Read the model definition and answer for the solid it produces. Units are mm, in the model's axes. A direction names the side the tool comes from. Coordinates: 2 decimals unless noted, no trailing zeros. Write each loop counter-clockwise with the first axis right and the second up, starting at its lowest first coordinate (ties: lowest second). Pieces come first, ordered by that corner, then holes.
(1) Which of the six approach directions +Z, -Z, +X, -X, +Y, -Y give full straight-line access (tool end or side, diameter ignored) to faces 4 (the flat face through (66.302, -3.639, 4.93)), 5 (the flat face through (-66.751, -3.898, 4.93)), 6 (the flat face through (-67.34, -39.36, 4.93))?
(2) Find the intervals of material crossed by probe 1 along Z at (x, y) = (59, 0); probe 2 along Y at (x, z) = (0, 7); probe 3 along Z at (x, y) = (-50, -10), in increasing order.
(3) Given pin 1 (12 mm diameter, centred on x = 25, z = 853.5, fed in from +Y); pin 2 (10 mm diameter, centred on y = 42.5, z = 256, fed in from -X); pin 3 (2 mm diameter, centred on x = 16, y = 53.5, fed in from +Z); pin 4 (1 mm diameter, centred on x = -12, y = 14, fed in from -Z), each flat-ended and moving along its own axis, determine where each tip first touches the part or whether it passes through.
(4) Section A-A on y = 25 is taken. Write down the section's boundary in (x, z), then the cut area to 3 significant figures.
(5) The mould has two halves that part along Z. Classify faces 1 (the flat face through (67.76, -38.64, 4.93)), 2 (the flat face through (-7, 5, 0)), 3 (the cylindrical face through (-57.887, -37.099, 1129.553)): +Z half, -Z half, draft (parallel to the pull), parting line (faces both ways), or undercut.
(6) Section B-B on z = 1074 is taken. Write down the section's boundary in (x, y).
Autodesk Inventor part; units mm, degrees
ref_plane "YZ Plane" through (0, 0, 0) normal (1, 0, 0) x (0, 1, 0)
ref_plane "XZ Plane" through (0, 0, 0) normal (0, 1, 0) x (-1, 0, 0)
ref_plane "XY Plane" through (0, 0, 0) normal (0, 0, 1) x (1, 0, 0)
sketch "Sketch1" plane through (0, 0, 0) normal (0, 0, 1) x (1, 0, 0)
  line L0 (-30, 78) -> (30, 78)
  line L1 (30, 78) -> (30, 8)
  line L2 (30, 8) -> (-30, 8)
  line L3 (-30, 8) -> (-30, 78)
  line L4 (119.0409, 377.068) -> (884.0572, 377.068) construction
  line L5 (884.0572, 377.068) -> (884.0572, -61.283) construction
  line L6 (884.0572, -61.283) -> (119.0409, -61.283) construction
  line L7 (119.0409, -61.283) -> (119.0409, 377.068) construction
  line L8 (528.2997, 310.003) -> (528.2997, 129.9198)
  line L9 (528.2997, 219.9614) -> (642.893, 286.807)
  circle A0 centre (0, 65) radius 6.5
  point P0 (0, 0)
  point P1 (0, 8)
  point P2 (0, 78)
  dimension "d9" = 60
  dimension "d10" = 70
  dimension "d13" = 78
  dimension "d14" = 13
  dimension "d15" = 13
extrude "Extrusion1" add sketch "Sketch1" along normal blind 10
pattern_circular "Circular Pattern1" count 3 over 360 about axis through (0, 0, -10) along (0, 0, 1) of "Extrusion1"
sketch "Sketch2" plane through (0, 0, 0) normal (0, 0, 1) x (1, 0, 0)
  circle A0 centre (0, 0) radius 50.8
  dimension "d21" = 101.6
extrude "Extrusion2" add sketch "Sketch2" along normal blind 1211
sketch "Sketch3" plane through (0, 0, 0) normal (1, 0, 0) x (0, 1, 0)
  circle A0 centre (0, 83) radius 48.75
  circle A1 centre (0, 83) radius 46.75
  point P0 (0, 0)
  dimension "d24" = 97.5
  dimension "d25" = 83
  dimension "d112" = 2
extrude "Extrusion3" add sketch "Sketch3" along normal blind 82.8
sketch "Sketch4" plane through (0, 0, 0) normal (1, 0, 0) x (0, 1, 0)
  circle A0 centre (0, 1158) radius 48.75
  line L0 (508.6061, 725.4056) -> (1697.4131, 725.4056) construction
  line L1 (1697.4131, 725.4056) -> (1697.4131, 178.9914) construction
  line L2 (1697.4131, 178.9914) -> (508.6061, 178.9914) construction
  line L3 (508.6061, 178.9914) -> (508.6061, 725.4056) construction
  line L4 (1437.8763, 515.5441) -> (1697.4131, 515.5441)
  line L5 (1697.4131, 515.5441) -> (1697.4131, 335.5441)
  line L6 (1697.4131, 335.5441) -> (1437.8763, 335.5441)
  line L7 (1437.8763, 335.5441) -> (1437.8763, 515.5441)
  line L8 (1526.1756, 486.7469) -> (1616.156, 486.7469)
  line L9 (40.9956, 0) -> (40.9956, 10)
  line L10 (40.9956, 0) -> (5.483, 0)
  line L11 (5.483, 10) -> (5.483, 0)
  line L12 (-46.4786, 10) -> (5.483, 10)
  line L13 (-46.4786, 0) -> (-46.4786, 10)
  line L14 (-46.4786, 0) -> (-46.4786, 0)
  line L15 (-46.4786, 10) -> (-46.4786, 0)
  line L16 (5.483, 10) -> (-46.4786, 10)
  line L17 (5.483, 0) -> (5.483, 10)
  line L18 (5.483, 0) -> (40.9956, 0)
  line L19 (40.9956, 10) -> (40.9956, 0)
  line L20 (40.9956, 10) -> (40.9956, 10)
  line L21 (50.8, 1211) -> (-50.8, 1211)
  circle A1 centre (0, 1158) radius 46.75
  line L22 (78, 0) -> (40.9956, 0)
  point P0 (0, 0)
  point P1 (48.75, 83)
  dimension "d28" = 97.5
  dimension "d71" = 180
  dimension "d90" = 89.9804
  dimension "d93" = 53
  dimension "d103" = 2
  dimension "d114" = 1158
extrude "Extrusion4" add sketch "Sketch4" against normal blind 82.8 contours A0
sketch "Sketch5" plane through (-82.8, 0, 1158) normal (-1, 0, 0) x (0, 0, 1)
  circle A0 centre (0, 0) radius 48.75
  circle A1 centre (0, 0) radius 110
  circle A2 centre (0, 0) radius 90 construction
  circle A3 centre (90, 0) radius 8
  circle A4 centre (63.6396, 63.6396) radius 8
  circle A5 centre (0, 90) radius 8
  circle A6 centre (-63.6396, 63.6396) radius 8
  circle A7 centre (-90, 0) radius 8
  circle A8 centre (-63.6396, -63.6396) radius 8
  circle A9 centre (0, -90) radius 8
  circle A10 centre (63.6396, -63.6396) radius 8
  point P0 (-1158, 0)
  dimension "d95" = 180
  dimension "d94" = 220
  dimension "d96" = 16
  dimension "d99" = 360
extrude "Extrusion5" [suppressed]
sketch "Sketch6" plane through (82.8, 0, 83) normal (1, 0, 0) x (0, 0, -1)
  circle A0 centre (0, 0) radius 110
  circle A1 centre (0, 0) radius 90 construction
  circle A2 centre (-90, 0) radius 8
  circle A3 centre (-63.6396, -63.6396) radius 8
  circle A4 centre (0, -90) radius 8
  circle A5 centre (63.6396, -63.6396) radius 8
  circle A6 centre (90, 0) radius 8
  circle A7 centre (63.6396, 63.6396) radius 8
  circle A8 centre (0, 90) radius 8
  circle A9 centre (-63.6396, 63.6396) radius 8
  circle A10 centre (0, 0) radius 48.75
  point P0 (83, 0)
  dimension "d107" = 180
  dimension "d106" = 220
  dimension "d108" = 16
  dimension "d109" = 360
extrude "Extrusion6" [suppressed]
equation "\"d21\" = main_diameter"
equation "\"d22\" = main_height"
equation "\"d24\" = connect_pipe"
equation "\"d28\" = connect_pipe"
equation "\"main_height\" = 1211"
equation "\"connect_pipe\" = 97.5"
equation "\"main_diameter\" = 101.6"
properties part number "UV-Cleaner ODV-15"
Response:
1. face 4: -Z, +X, +Y
1. face 5: -Z, -X, +Y
1. face 6: -Z, -X, -Y
2. probe 1: z = 0 to 10, 34.25 to 36.25, 129.75 to 131.75
2. probe 2: y = -50.8 to 58.5, 71.5 to 78
2. probe 3: z = 0 to 10, 1110.29 to 1112.33, 1203.67 to 1205.71
3. pin 1: stops at y = 47.11
3. pin 2: stops at x = -34.27
3. pin 3: stops at z = 10
3. pin 4: stops at z = 0
4. outline: (-82.8, 1116.15) - (-44.22, 1116.15) - (-44.22, 0) - (44.22, 0) - (44.22, 41.15) - (82.8, 41.15) - (82.8, 43.5) - (44.22, 43.5) - (44.22, 122.5) - (82.8, 122.5) - (82.8, 124.85) - (44.22, 124.85) - (44.22, 1211) - (-44.22, 1211) - (-44.22, 1199.85) - (-82.8, 1199.85) - (-82.8, 1197.5) - (-44.22, 1197.5) - (-44.22, 1118.5) - (-82.8, 1118.5) - close
4. area: 107,000 mm2
5. face 1: draft
5. face 2: -Z half
5. face 3: undercut
6. outline: circle Ø101.6 at (0, 0)
